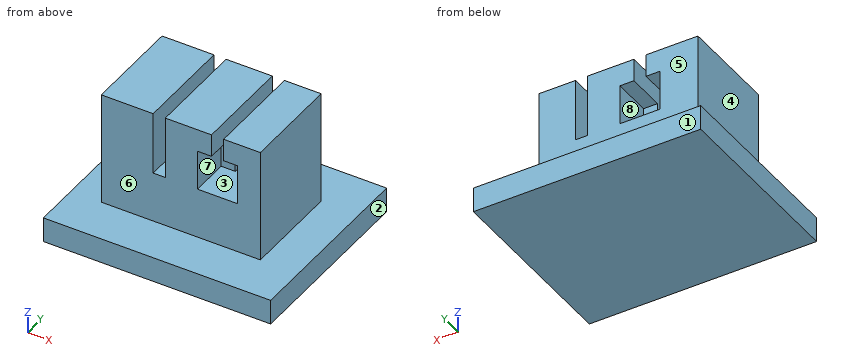
```python
from build123d import *

# Parameters (mm, degrees)
F0_W      = 30
F0_H      = 25
F1_DEPTH  = 3.3
F2_W      = 21
F2_H      = 13.1
F3_DEPTH  = 15
F4_W      = 5.3
F4_H      = 5.3
F5_DEPTH  = 5.1
F6_W      = 1.6
F6_H      = 13.1
F7_DEPTH  = 8.3
F8_W      = 5.3
F8_H      = 5.3
F9_DEPTH  = 5.1
F10_W     = 1.6
F10_H     = 13.1
F11_DEPTH = 8.3


# Not quite as in the source:
# - a feature names something its author has since deleted; it is built from what else it names


with BuildPart() as f1:
    # F0 (on Top) → F1 (new body)
    with BuildSketch(Plane.XY):
        Rectangle(F0_W, F0_H)
    extrude(amount=F1_DEPTH)

    # F2 (on face) → F3 (join)
    with BuildSketch(Plane.XY.offset(3.3)):
        with Locations((-0.5, 0)):
            Rectangle(F2_W, F2_H)
    extrude(amount=F3_DEPTH)

    # F4 (on face) → F5 (cut)
    with BuildSketch(Plane.XZ.offset(6.55)):
        with Locations((4.35, 12.65)):
            Rectangle(F4_W, F4_H)
    extrude(amount=-F5_DEPTH, mode=Mode.SUBTRACT)

    # F6 (on face) → F7 (cut)
    with BuildSketch(Plane.XY.offset(18.3)):
        with Locations((4.35, 0)):
            Rectangle(F6_W, F6_H)
    extrude(amount=-F7_DEPTH, mode=Mode.SUBTRACT)

    # F8 (on face) → F9 (cut)
    with BuildSketch(Plane(origin=(0, 6.55, 0), x_dir=(-1, 0, 0), z_dir=(0, 1, 0))):
        with Locations((3.35, 12.65)):
            Rectangle(F8_W, F8_H)
    extrude(amount=-F9_DEPTH, mode=Mode.SUBTRACT)

    # F10 (on face) → F11 (cut)
    with BuildSketch(Plane.XY.offset(18.3)):
        with Locations((-3.35, 0)):
            Rectangle(F10_W, F10_H)
    extrude(amount=-F11_DEPTH, mode=Mode.SUBTRACT)


solid = f1.part
```
Model file for the job. Use its own axes, mm. Face numbers are marked on the shaded views. A direction names the side the tool comes from. Round coordinates to 2 decimals unless told otherwise and drop trailing zeros. Write each loop counter-clockwise with the first axis right and the second up, starting at its lowest first coordinate (ties: lowest second). Pieces come first, ordered by that corner, then holes. Notation, with made-up numbers: (16, -20) - (53, -20) arc R32 ccw to (53, 18) - close; hole circle Ø4 at (36.5, 35.5). An arc over 180 degrees is marked (long way). Use CSV: the item, a comma, the result in double quotes. Start each with the question number.
Item 1: Two-plate mould, pull along X, no slides. Class the marked faces 1, 2 and 3: released by +X, released by -X, zero draft, split by the parting line, or undercut.
Item 2: Band-saw the part on B-B (y = 3.75). Write the cut outline in (x, z).
Item 3: Pin check, flat tips, straight feed: P1, Ø1, axis at y = -6.5, z = 9, coming from the +X side; P2, Ø3, axis at x = -7, z = 14.5, coming from the -Y side; P3, Ø1.5, axis at y = 4.5, z = 12.5, coming from the -X side. Stop position of each tip, or through.
Item 4: Tool access for the marked faces 4, 5, 6, 7 and 8: list every direction of +Z, -Z, +X, -X, +Y, -Y with a clear straight run to the whole face (end or side of a thin tool).
Item 5: Band-saw the part on C-C (x = 3). Write the cut outline in (y, z).
Item 6: Band-saw the part on A-A (z = 13). Write the cut outline in (x, y).
Item 7: Drill centre lines: L1, parallel to X at y = 2, z = 16; L2, parallel to Z at x = 3.5, y = 10; L3, parallel to X at y = -2.5, z = 6. Where is each one in solid material? Low to high. Write a range as [from, to].
Item 8: Band-saw the part on D-D (x = -0.25). Write the cut outline in (y, z).
Checked values:
1,face 1,"zero draft"
1,face 2,"released by +X"
1,face 3,"undercut"
2,outline,"(-15, 0) - (15, 0) - (15, 3.3) - (10, 3.3) - (10, 18.3) - (5.15, 18.3) - (5.15, 10) - (3.55, 10) - (3.55, 18.3) - (-2.55, 18.3) - (-2.55, 15.3) - (-0.7, 15.3) - (-0.7, 10) - (-6, 10) - (-6, 15.3) - (-4.15, 15.3) - (-4.15, 18.3) - (-11, 18.3) - (-11, 3.3) - (-15, 3.3) - close"
3,P1,"stops at x = 10"
3,P2,"stops at y = -6.55"
3,P3,"stops at x = -11"
4,face 4,"+Z, -X, +Y, -Y"
4,face 5,"+Z, +X, -X, +Y"
4,face 6,"+Z, +X, -X, -Y"
4,face 7,"-Y"
4,face 8,"+Y"
5,outline,"(-12.5, 0) - (12.5, 0) - (12.5, 3.3) - (6.55, 3.3) - (6.55, 18.3) - (-6.55, 18.3) - (-6.55, 15.3) - (-1.45, 15.3) - (-1.45, 10) - (-6.55, 10) - (-6.55, 3.3) - (-12.5, 3.3) - close"
6,outline,"(-11, -6.55) - (-4.15, -6.55) - (-4.15, 1.45) - (-6, 1.45) - (-6, 6.55) - (-11, 6.55) - close; (-2.55, -6.55) - (1.7, -6.55) - (1.7, -1.45) - (3.55, -1.45) - (3.55, 6.55) - (-0.7, 6.55) - (-0.7, 1.45) - (-2.55, 1.45) - close; (5.15, -1.45) - (7, -1.45) - (7, -6.55) - (10, -6.55) - (10, 6.55) - (5.15, 6.55) - close"
7,L1,"x = [-11, -4.15], [-2.55, 3.55], [5.15, 10]"
7,L2,"z = [0, 3.3]"
7,L3,"x = [-11, 10]"
8,outline,"(-12.5, 0) - (12.5, 0) - (12.5, 3.3) - (6.55, 3.3) - (6.55, 18.3) - (-6.55, 18.3) - (-6.55, 3.3) - (-12.5, 3.3) - close"
